from build123d import *

# Parameters (mm, degrees)
BOSS_EXTRUDE1_DEPTH   = 4
SKETCH4_W             = 71.532637276
SKETCH4_H             = 26.364466528
CUT_EXTRUDE1_DEPTH    = 4
F_4_0MM_DOWEL_HOLE1_D = 4


with BuildPart() as part:
    # Sketch1 → Boss-Extrude1 (new body)
    with BuildSketch(Plane(origin=(0, 0, 0), x_dir=(1, 0, 0), z_dir=(0, 1, 0))):
        with BuildLine():
            Line((-148.5, -110), (148.5, -110))
            ThreePointArc((148.5, -110), (152.035533906, -108.535533906), (153.5, -105))
            Line((153.5, -105), (153.5, 105))
            ThreePointArc((153.5, 105), (152.035533906, 108.535533906), (148.5, 110))
            Line((148.5, 110), (-148.5, 110))
            ThreePointArc((-148.5, 110), (-152.035533906, 108.535533906), (-153.5, 105))
            Line((-153.5, 105), (-153.5, -105))
            ThreePointArc((-153.5, -105), (-152.035533906, -108.535533906), (-148.5, -110))
        make_face()
    extrude(amount=BOSS_EXTRUDE1_DEPTH)

    # Sketch4 → Cut-Extrude1 (cut)
    with BuildSketch(Plane(origin=(0, 4, 0), x_dir=(1, 0, 0), z_dir=(0, 1, 0))):
        Polygon((-153.5, 10.290131999), (-80.023243562, 10.290131999), (-80.023243562, 7.383174491), (-76.226434875, 3.638376882), (-76.226434875, -30.63211249), (-79.068246362, -33.513393581), (-79.068246362, -47.279961532), (-153.5, -47.279961532), align=None)
        with Locations((32.833027244, 50.697784315)):
            Rectangle(SKETCH4_W, SKETCH4_H)
        with BuildLine():
            Line((108.837010637, 57.559292177), (114.585798826, 57.559292177))
            ThreePointArc((114.585798826, 57.559292177), (118.121332732, 56.094826083), (119.585798826, 52.559292177))
            Line((119.585798826, 52.559292177), (119.585798826, 38.593744934))
            ThreePointArc((119.585798826, 38.593744934), (118.121332732, 35.058211028), (114.585798826, 33.593744934))
            Line((114.585798826, 33.593744934), (108.837010637, 33.593744934))
            ThreePointArc((108.837010637, 33.593744934), (105.301476732, 35.058211028), (103.837010637, 38.593744934))
            Line((103.837010637, 38.593744934), (103.837010637, 52.559292177))
            ThreePointArc((103.837010637, 52.559292177), (105.301476732, 56.094826083), (108.837010637, 57.559292177))
        make_face()
        with BuildLine():
            Line((-13.526451363, -56.423479831), (101.946204315, -56.423479831))
            ThreePointArc((101.946204315, -56.423479831), (105.481738221, -57.887945925), (106.946204315, -61.423479831))
            Line((106.946204315, -61.423479831), (106.946204315, -68.367080563))
            ThreePointArc((106.946204315, -68.367080563), (105.481738221, -71.902614469), (101.946204315, -73.367080563))
            Line((101.946204315, -73.367080563), (-13.526451363, -73.367080563))
            ThreePointArc((-13.526451363, -73.367080563), (-17.061985269, -71.902614469), (-18.526451363, -68.367080563))
            Line((-18.526451363, -68.367080563), (-18.526451363, -61.423479831))
            ThreePointArc((-18.526451363, -61.423479831), (-17.061985269, -57.887945925), (-13.526451363, -56.423479831))
        make_face()
    extrude(amount=-CUT_EXTRUDE1_DEPTH, mode=Mode.SUBTRACT)

    # Ø4.0mm Dowel Hole1 (through all)
    with Locations(Plane(origin=(0, 4, 0), x_dir=(1, 0, 0), z_dir=(0, 1, 0))):
        with Locations((-141, -97.5000082), (140.9999974, -97.5000082), (141, 97.5), (-141, 97.5)):
            Hole(F_4_0MM_DOWEL_HOLE1_D / 2)


solid = part.part
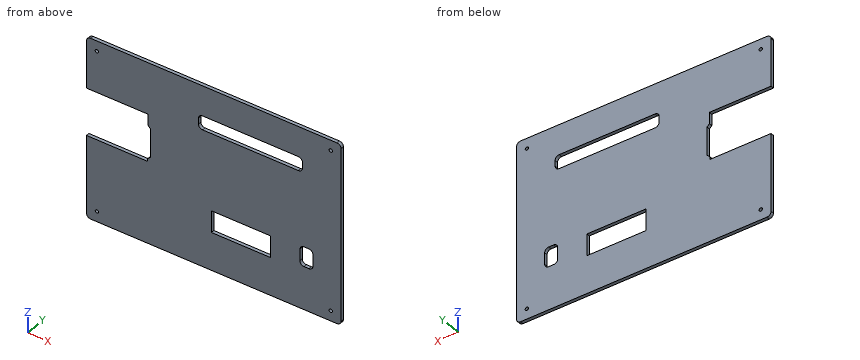
For this review, take the finished solid that the model builds, in its own axes (mm). Round coordinates to 2 decimals unless told otherwise and drop trailing zeros. Write each loop counter-clockwise with the first axis right and the second up, starting at its lowest first coordinate (ties: lowest second). Pieces come first, ordered by that corner, then holes. Notation, with made-up numbers: M 33,-12.5 L 86,-12.5 A9 ccw 86,3.5 Z; hole C 12,76.25 d11. An arc over 180 degrees is marked long. Write item = value, one per line. Start each with the question number.
(1) For line 1 along Z through (x, y) = (11, 3.45); line 2 along X through (y, z) = (0.8, -97.5); line 3 along Z through (x, y) = (-141, 1.5), list the stretches that pass through material, from the lowest coordinate up.
(2) Clearance check with a flat-ended pin moving along its axis: pin 1 Ø2.5 at (x, z) = (141, -97.5) entering from -Y. State where the tip first meets the part, or that it passes through.
(3) We need section D-D (z = 44). Give the boundary of the cut face in (x, y), then the cut area to 3 significant figures.
(4) We need section B-B (x = -126.5). Give the boundary of the cut face in (y, z), then the cut area to 3 significant figures.
(5) We need section C-C (y = 1.65). Give the number of separate pieces and of enclosed holes in the cut face, then the cut area to 3 significant figures.
(6) We need section A-A (x = 62.5). Give the boundary of the cut face in (y, z), then the cut area to 3 significant figures.
Results found:
q1.line_1 = -110 to -63.88, -37.52 to 56.42, 73.37 to 110
q1.line_2 = -153.5 to -143, -139 to 139, 143 to 153.5
q1.line_3 = -110 to -99.5, -95.5 to -10.29, 47.28 to 95.5, 99.5 to 110
q2.pin_1 = through
q3.outline = M -79.07,0 L 153.5,0 L 153.5,4 L -79.07,4 Z
q3.area = 930 mm²
q4.outline = M 0,-110 L 4,-110 L 4,-10.29 L 0,-10.29 Z; M 0,47.28 L 4,47.28 L 4,110 L 0,110 Z
q4.area = 650 mm²
q5.separate_pieces = 1
q5.enclosed_holes = 7
q5.area = 58,700 mm²
q6.outline = M 0,-110 L 4,-110 L 4,-63.88 L 0,-63.88 Z; M 0,-37.52 L 4,-37.52 L 4,56.42 L 0,56.42 Z; M 0,73.37 L 4,73.37 L 4,110 L 0,110 Z
q6.area = 707 mm²
